```python
from build123d import *

# Parameters (mm, degrees)
SKETCH1_R           = 2.4384
BOSS_EXTRUDE1_DEPTH = 3.175
FILLET3_R           = 5.08


with BuildPart() as part:
    # Sketch1 → Boss-Extrude1 (new body)
    with BuildSketch(Plane(origin=(0, 0, 0), x_dir=(1, 0, 0), z_dir=(0, 1, 0))):
        with BuildLine():
            ThreePointArc((5.08, 0), (1.487897552, -1.487897552), (0, -5.08))
            Line((0, -5.08), (0, -71.12))
            ThreePointArc((0, -71.12), (1.487897552, -74.712102448), (5.08, -76.2))
            Line((5.08, -76.2), (25.4, -76.2))
            Line((25.4, -76.2), (72.39, -50.8))
            Line((72.39, -50.8), (72.39, 0))
            Line((72.39, 0), (5.08, 0))
        make_face()
        with Locations(Location((50.8, -38.1, 0), (0, 0, 270))):
            Circle(SKETCH1_R, mode=Mode.SUBTRACT)
        with Locations(Location((50.8, -25.4, 0), (0, 0, 270))):
            Circle(SKETCH1_R, mode=Mode.SUBTRACT)
        with Locations(Location((50.8, -12.7, 0), (0, 0, 270))):
            Circle(SKETCH1_R, mode=Mode.SUBTRACT)
        with Locations(Location((12.7, -63.5, 0), (0, 0, 270))):
            Circle(SKETCH1_R, mode=Mode.SUBTRACT)
        with Locations(Location((63.5, -38.1, 0), (0, 0, 270))):
            Circle(SKETCH1_R, mode=Mode.SUBTRACT)
        with Locations(Location((63.5, -25.4, 0), (0, 0, 270))):
            Circle(SKETCH1_R, mode=Mode.SUBTRACT)
        with Locations(Location((63.5, -12.7, 0), (0, 0, 270))):
            Circle(SKETCH1_R, mode=Mode.SUBTRACT)
        with Locations(Location((12.7, -38.1, 0), (0, 0, 270))):
            Circle(SKETCH1_R, mode=Mode.SUBTRACT)
        with Locations(Location((12.7, -12.7, 0), (0, 0, 270))):
            Circle(SKETCH1_R, mode=Mode.SUBTRACT)
        with Locations(Location((38.1, -38.1, 0), (0, 0, 270))):
            Circle(SKETCH1_R, mode=Mode.SUBTRACT)
        with Locations(Location((38.1, -25.4, 0), (0, 0, 270))):
            Circle(SKETCH1_R, mode=Mode.SUBTRACT)
        with Locations(Location((38.1, -12.7, 0), (0, 0, 270))):
            Circle(SKETCH1_R, mode=Mode.SUBTRACT)
    extrude(amount=BOSS_EXTRUDE1_DEPTH)

    # Fillet3
    fillet3_edges = [part.edges().sort_by_distance(p)[0] for p in [
        (72.39, 1.5875, 0),
        (72.39, 1.5875, 50.8),
        (25.4, 1.5875, 76.2),
    ]]
    fillet(fillet3_edges, radius=FILLET3_R)


solid = part.part
```
Geometry: final body of the model. Coordinates: model frame, mm. Round coordinates to 2 decimals unless told otherwise and drop trailing zeros. Write each loop counter-clockwise with the first axis right and the second up, starting at its lowest first coordinate (ties: lowest second). Pieces come first, ordered by that corner, then holes. Notation, with made-up numbers: (6.5, -39.75) -> (19.5, -39.75) arc R29 cw to (19.5, -3.75) -> close; hole circle Ø6 at (62, 6). An arc over 180 degrees is marked (long way). Return JSON: item names as keys, results as strings.
Q1. First-contact query: pin 1 Ø1.5 at (y, z) = (0.5, 59) entering from +X. Flat tip, straight axial feed; report the tip coordinate or a pass-through.
From the geometry:
{"pin 1": "x = 58.61"}
Q2. Section D-D on y = 1.55. Give the number of separate pieces and of enclosed holes in the cut face, and give its area (3 significant figures).
From the geometry:
{"separate pieces": "1", "enclosed holes": "12", "area": "4,680 mm2"}
Q3. Mould query, pull axis Z, two halves, no side actions, for faces 1 (the cylindrical face through (10.54, 1.57, 13.83)), 2 (the flat face through (47.826, 1.565, 64.078)), 3 (the cylindrical face through (51.532, 1.565, 15.026)), 4 (the cylindrical face through (70.862, 1.61, 1.449)). Classes: +Z half, -Z half, draft (parallel to the pull), parting line (faces both ways), or undercut.
From the geometry:
{"face 1": "undercut", "face 2": "+Z half", "face 3": "undercut", "face 4": "-Z half"}
Q4. Section B-B on x = 63.5. Return the cut outline in (y, z) (3 decimals), and give its area (3 significant figures).
From the geometry:
{"outline": "(0, 0) -> (3.175, 0) -> (3.175, 10.262) -> (0, 10.262) -> close; (0, 15.138) -> (3.175, 15.138) -> (3.175, 22.962) -> (0, 22.962) -> close; (0, 27.838) -> (3.175, 27.838) -> (3.175, 35.662) -> (0, 35.662) -> close; (0, 40.538) -> (3.175, 40.538) -> (3.175, 55.605) -> (0, 55.605) -> close", "area": "130 mm2"}
Q5. Ray query, line 1 (X direction, y = 1.3, z = 25.4); line 2 (Z direction, x = 12.5, y = 1.5); line 3 (X direction, y = 2.55, z = 38). Return the intervals inside material, ascending.
From the geometry:
{"line 1": "0 to 35.66, 40.54 to 48.36, 53.24 to 61.06, 65.94 to 72.39", "line 2": "0 to 10.27, 15.13 to 35.67, 40.53 to 61.07, 65.93 to 76.2", "line 3": "0 to 10.26, 15.14 to 35.66, 40.54 to 48.36, 53.24 to 61.06, 65.94 to 72.39"}
Q6. Section A-A on z = 25.4. Return the cut outline in (x, y) (3 decimals).
From the geometry:
{"outline": "(0, 0) -> (35.662, 0) -> (35.662, 3.175) -> (0, 3.175) -> close; (40.538, 0) -> (48.362, 0) -> (48.362, 3.175) -> (40.538, 3.175) -> close; (53.238, 0) -> (61.062, 0) -> (61.062, 3.175) -> (53.238, 3.175) -> close; (65.938, 0) -> (72.39, 0) -> (72.39, 3.175) -> (65.938, 3.175) -> close"}
Q7. Section C-C on z = 12.7. Return the cut outline in (x, y) (3 decimals).
From the geometry:
{"outline": "(0, 0) -> (10.262, 0) -> (10.262, 3.175) -> (0, 3.175) -> close; (15.138, 0) -> (35.662, 0) -> (35.662, 3.175) -> (15.138, 3.175) -> close; (40.538, 0) -> (48.362, 0) -> (48.362, 3.175) -> (40.538, 3.175) -> close; (53.238, 0) -> (61.062, 0) -> (61.062, 3.175) -> (53.238, 3.175) -> close; (65.938, 0) -> (72.39, 0) -> (72.39, 3.175) -> (65.938, 3.175) -> close"}
